Input: part model. Units: mm. Frame: model coordinates. A direction names the side the tool comes from. Round coordinates to 2 decimals unless told otherwise and drop trailing zeros. Loops run counter-clockwise (first coordinate to the right, second up) from the corner with the lowest first, then second, coordinate; pieces in that order, holes last. Notation, with made-up numbers: (54.25, 78.5) -> (110.25, 78.5) arc R13 cw to (110.25, 88.5) -> close; hole circle Ø6 at (30, 65). An arc over 180 degrees is marked (long way). Answer as a JSON object with one key per item and string values. Group by question number.
Item 1: Material intervals for line 1 (X direction, y = 1, z = 10.25); line 2 (X direction, y = 1.05, z = -10.1); line 3 (Z direction, x = 9.25, y = 1), sorted ascending. Write a range as [from, to].
Item 2: Section query B-B on x = -5.25. Return loops of the section in (y, z).
Item 3: Section query D-D on x = -11. Return loops of the section in (y, z).
Item 4: Section query A-A on z = -4. Return loops of the section in (x, y) (3 decimals), and give its area (3 significant figures).
Item 5: Pin query (flat end, axial travel): pin 1 (1.5 mm diameter, centred on x = -6.5, y = 8.5, fed in from +Z). Return the tip coordinate at first contact, or that it passes through.
Item 6: Section query C-C on y = 1.25. Return loops of the section in (x, z).
Item 7: Set-up query: faces 1 (the flat face through (12, 3, 6)), 2 (the flat face through (-12, 3, 6)), 3 (the flat face through (-7.7, 6.45, 11.02)), 4 (the cylindrical face through (0.1, 6.5, -12.5)), 5 (the flat face through (-12.5, 1, 0)). Return all of +Z, -Z, +X, -X, +Y, -Y with unobstructed straight access to the full face (end or side cutting, diameter ignored); none if empty.
Item 8: Draft query along Z for faces 6 (the flat face through (0, 1, 12.5)), 7 (the flat face through (12, 3, -6)), 8 (the flat face through (-9.32, 0, 7.35)). Return one class per face: released by +Z, released by -Z, zero draft, split by the parting line, or undercut.
from build123d import *

# Parameters (mm, degrees)
SKETCH_1_R          = 11.7
EXTRUDE_1_DEPTH     = 3
SKETCH_2_R          = 1.25
SKETCH_2_R_2        = 11.7
EXTRUDE_2_DEPTH     = 7
SKETCH_2_3_R        = 1.25
CUT_EXTRUDE_1_DEPTH = 20.013153342


with BuildPart() as part:
    # Sketch 1 → Extrude 1 (new body)
    with BuildSketch(Plane(origin=(0, 0, 0), x_dir=(1, 0, 0), z_dir=(0, 1, 0))):
        with BuildLine():
            Line((-10.1, -12.5), (10.1, -12.5))
            ThreePointArc((10.1, -12.5), (11.797056275, -11.797056275), (12.5, -10.1))
            Line((12.5, -10.1), (12.5, 10.1))
            ThreePointArc((12.5, 10.1), (11.797056275, 11.797056275), (10.1, 12.5))
            Line((10.1, 12.5), (-10.1, 12.5))
            ThreePointArc((-10.1, 12.5), (-11.797056275, 11.797056275), (-12.5, 10.1))
            Line((-12.5, 10.1), (-12.5, -10.1))
            ThreePointArc((-12.5, -10.1), (-11.797056275, -11.797056275), (-10.1, -12.5))
        make_face()
        with Locations(Location((0, 0, 0), (0, 0, 270))):
            Circle(SKETCH_1_R, mode=Mode.SUBTRACT)
    extrude(amount=EXTRUDE_1_DEPTH)

    # Sketch 2 → Extrude 2 (add)
    with BuildSketch(Plane(origin=(0, 3, 0), x_dir=(1, 0, 0), z_dir=(0, 1, 0))):
        with BuildLine():
            ThreePointArc((-7.067198742, -10.310417156), (0, -12.5), (7.067198742, -10.310417156))
            Line((7.067198742, -10.310417156), (8.311827358, -11.700761882))
            ThreePointArc((8.311827358, -11.700761882), (9.12067077, -12.29109887), (10.1, -12.5))
            ThreePointArc((10.1, -12.5), (11.797056275, -11.797056275), (12.5, -10.1))
            ThreePointArc((12.5, -10.1), (12.29109887, -9.12067077), (11.700761882, -8.311827358))
            Line((11.700761882, -8.311827358), (10.310417156, -7.067198742))
            ThreePointArc((10.310417156, -7.067198742), (12.5, 0), (10.310417156, 7.067198742))
            Line((10.310417156, 7.067198742), (11.700761882, 8.311827358))
            ThreePointArc((11.700761882, 8.311827358), (12.29109887, 9.12067077), (12.5, 10.1))
            ThreePointArc((12.5, 10.1), (11.797056275, 11.797056275), (10.1, 12.5))
            ThreePointArc((10.1, 12.5), (9.12067077, 12.29109887), (8.311827358, 11.700761882))
            Line((8.311827358, 11.700761882), (7.067198742, 10.310417156))
            ThreePointArc((7.067198742, 10.310417156), (0, 12.5), (-7.067198742, 10.310417156))
            Line((-7.067198742, 10.310417156), (-8.311827358, 11.700761882))
            ThreePointArc((-8.311827358, 11.700761882), (-9.12067077, 12.29109887), (-10.1, 12.5))
            ThreePointArc((-10.1, 12.5), (-11.797056275, 11.797056275), (-12.5, 10.1))
            ThreePointArc((-12.5, 10.1), (-12.29109887, 9.12067077), (-11.700761882, 8.311827358))
            Line((-11.700761882, 8.311827358), (-10.310417156, 7.067198742))
            ThreePointArc((-10.310417156, 7.067198742), (-12.5, 0), (-10.310417156, -7.067198742))
            Line((-10.310417156, -7.067198742), (-11.700761882, -8.311827358))
            ThreePointArc((-11.700761882, -8.311827358), (-12.29109887, -9.12067077), (-12.5, -10.1))
            ThreePointArc((-12.5, -10.1), (-11.797056275, -11.797056275), (-10.1, -12.5))
            ThreePointArc((-10.1, -12.5), (-9.12067077, -12.29109887), (-8.311827358, -11.700761882))
            Line((-8.311827358, -11.700761882), (-7.067198742, -10.310417156))
        make_face()
        with Locations(Location((-10.1, -10.1, 0), (0, 0, 270))):
            Circle(SKETCH_2_R, mode=Mode.SUBTRACT)
        with Locations(Location((10.1, -10.1, 0), (0, 0, 270))):
            Circle(SKETCH_2_R, mode=Mode.SUBTRACT)
        with Locations(Location((10.1, 10.1, 0), (0, 0, 270))):
            Circle(SKETCH_2_R, mode=Mode.SUBTRACT)
        with Locations(Location((-10.1, 10.1, 0), (0, 0, 270))):
            Circle(SKETCH_2_R, mode=Mode.SUBTRACT)
        with Locations(Location((0, 0, 0), (0, 0, 270))):
            Circle(SKETCH_2_R_2, mode=Mode.SUBTRACT)
    extrude(amount=EXTRUDE_2_DEPTH)

    # Sketch 2_3 → Cut-Extrude 1 (cut, through all)
    with BuildSketch(Plane(origin=(0, 3, 0), x_dir=(1, 0, 0), z_dir=(0, 1, 0))):
        with Locations(Location((-10.1, 10.1, 0), (0, 0, 270))):
            Circle(SKETCH_2_3_R)
        with Locations(Location((10.1, 10.1, 0), (0, 0, 270))):
            Circle(SKETCH_2_3_R)
        with Locations(Location((10.1, -10.1, 0), (0, 0, 270))):
            Circle(SKETCH_2_3_R)
        with Locations(Location((-10.1, -10.1, 0), (0, 0, 270))):
            Circle(SKETCH_2_3_R)
    extrude(amount=-CUT_EXTRUDE_1_DEPTH, mode=Mode.SUBTRACT)


solid = part.part
Solved:
{
 "1": {"line 1": "[-12.5, -11.34], [-8.86, -5.64], [5.64, 8.86], [11.34, 12.5]", "line 2": "[-12.5, -11.35], [-8.85, -5.91], [5.91, 8.85], [11.35, 12.5]", "line 3": "[-12.5, -11.02], [-9.18, -7.16], [7.16, 9.18], [11.02, 12.5]"},
 "2": {"outline": "(0, -12.5) -> (3, -12.5) -> (3, -11.34) -> (10, -11.34) -> (10, -10.46) -> (0, -10.46) -> close; (0, 10.46) -> (10, 10.46) -> (10, 11.34) -> (3, 11.34) -> (3, 12.5) -> (0, 12.5) -> close"},
 "3": {"outline": "(0, -12.32) -> (10, -12.32) -> (10, -10.97) -> (0, -10.97) -> close; (0, -9.23) -> (10, -9.23) -> (10, -7.68) -> (3, -7.68) -> (3, -5.94) -> (10, -5.94) -> (10, -3.99) -> (0, -3.99) -> close; (0, 3.99) -> (10, 3.99) -> (10, 5.94) -> (3, 5.94) -> (3, 7.68) -> (10, 7.68) -> (10, 9.23) -> (0, 9.23) -> close; (0, 10.97) -> (10, 10.97) -> (10, 12.32) -> (0, 12.32) -> close"},
 "4": {"outline": "(-12.5, 0) -> (-10.995, 0) -> (-10.995, 10) -> (-11.843, 10) -> (-11.843, 3) -> (-12.5, 3) -> close; (10.995, 0) -> (12.5, 0) -> (12.5, 3) -> (11.843, 3) -> (11.843, 10) -> (10.995, 10) -> close", "area": "20.9 mm²"},
 "5": {"pin 1": "z = 11.1"},
 "6": {"outline": "(-12.5, -10.1) arc R2.4 ccw to (-10.1, -12.5) -> (10.1, -12.5) arc R2.4 ccw to (12.5, -10.1) -> (12.5, 10.1) arc R2.4 ccw to (10.1, 12.5) -> (-10.1, 12.5) arc R2.4 ccw to (-12.5, 10.1) -> close; hole circle Ø23.4 at (0, 0); hole circle Ø2.5 at (-10.1, -10.1); hole circle Ø2.5 at (-10.1, 10.1); hole circle Ø2.5 at (10.1, -10.1); hole circle Ø2.5 at (10.1, 10.1)"},
 "7": {"face 1": "+X, +Y", "face 2": "-X, +Y", "face 3": "+Z, +Y", "face 4": "-Z, +Y", "face 5": "+Z, -Z, -X, +Y, -Y"},
 "8": {"face 6": "released by +Z", "face 7": "undercut", "face 8": "zero draft"}
}
